Here's the drawing with two shaded views (mm, measured from the low corner). I have some questions. A direction names the side the tool comes from. Round coordinates to 2 decimals unless told otherwise and drop trailing zeros. Loops run counter-clockwise (first coordinate to the right, second up) from the corner with the lowest first, then second, coordinate; pieces in that order, holes last.
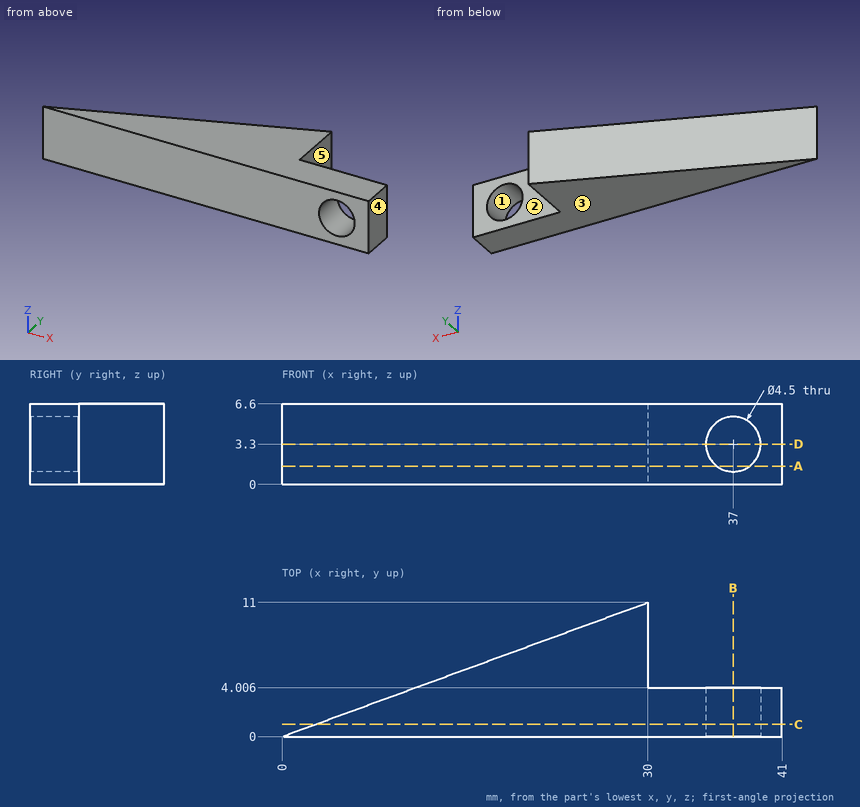
(1) If we section it at A-A, the plane z = 1.5: List the corners of the cut face in (x, y) for me.
Worked answers:
outline: (0, 0) - (35.65, 0) - (35.65, 4.01) - (30, 4.01) - (30, 11) - close; (38.35, 0) - (41, 0) - (41, 4.01) - (38.35, 4.01) - close
(2) If we section it at D-D, the plane z = 3.3: List the corners of the cut face in (x, y) for me, then the cut area to 3 significant figures.
Worked answers:
outline: (0, 0) - (34.75, 0) - (34.75, 4.01) - (30, 4.01) - (30, 11) - close; (39.25, 0) - (41, 0) - (41, 4.01) - (39.25, 4.01) - close
area: 191 mm2
(3) Will these pins go through, and if not, where does the flat tip stop? P1, Ø3.5, axis at y = 6.5, z = 3, coming from the +X side; P2, Ø1.5, axis at x = 4.5, z = 6, coming from the +Y side (3 decimals).
Worked answers:
P1: stops at x = 30
P2: stops at y = 1.925
(4) If we section it at C-C, the plane y = 1: List the corners of the cut face in (x, z) for me, then the cut area to 3 significant figures.
Worked answers:
outline: (2.73, 0) - (41, 0) - (41, 6.6) - (2.73, 6.6) - close; hole circle Ø4.5 at (37, 3.3)
area: 237 mm2
(5) If I drill on line 1 (Z direction, x = 37, y = 1.75); line 2 (Y direction, x = 31.5, z = 5.75); line 3 (Y direction, x = 7.5, z = 4.75), over which ranges is the centre line in solid material (lowest first)?
Worked answers:
line 1: z = 0 to 1.05, 5.55 to 6.6
line 2: y = 0 to 4.01
line 3: y = 0 to 2.75
(6) If we mould it in two halves opening along Z, with no side actions, what happens to the marked faces 1, 2 and 3? For each: released by +Z, released by -Z, zero draft, split by the parting line, or undercut.
Worked answers:
face 1: undercut
face 2: zero draft
face 3: released by -Z
(7) For the marked faces 4 and 5, which set-ups out of +Z, -Z, +X, -X, +Y, -Y let a thin tool reach every point of the face, with its end or its side?
Worked answers:
face 4: +Z, -Z, +X, +Y, -Y
face 5: +Z, -Z, +X, +Y
(8) If we section it at B-B, the plane x = 37: List the corners of the cut face in (y, z) for me.
Worked answers:
outline: (0, 0) - (4.01, 0) - (4.01, 1.05) - (0, 1.05) - close; (0, 5.55) - (4.01, 5.55) - (4.01, 6.6) - (0, 6.6) - close
